```python
from build123d import *

# Parameters (mm, degrees)
F1_DEPTH = 203.2
F2_R     = 3.69316
F3_R     = 1.98374
F4_R     = 0.762
F5_R     = 1.35255
F6_DEPTH = 1.70942


with BuildPart() as f1:
    # F0 (on Top) → F1 (new body)
    with BuildSketch(Plane.XY):
        Polygon((0, -34.912743), (0, 0), (4.632677, 3.932751), (7.97125, 0), (9.274422, 1.106282), (4.829567, 6.342205), (-1.70942, 0.791159), (-1.70942, -36.622163), (155.970525, -36.622163), (155.970525, 0.791159), (149.431538, 6.342205), (144.986683, 1.106282), (146.289855, 0), (149.628427, 3.932751), (154.261105, 0), (154.261105, -34.912743), align=None)
    extrude(amount=F1_DEPTH)

    # F2
    f2_edges = [f1.edges().sort_by_distance(p)[0] for p in [
        (149.431538, 6.342205, 101.6),
        (155.970525, 0.791159, 101.6),
        (155.970525, -36.622163, 101.6),
        (-1.70942, -36.622163, 101.6),
        (-1.70942, 0.791159, 101.6),
        (4.829567, 6.342205, 101.6),
    ]]
    fillet(f2_edges, radius=F2_R)

    # F3
    f3_edges = [f1.edges().sort_by_distance(p)[0] for p in [
        (149.628427, 3.932751, 101.6),
        (154.261105, 0, 101.6),
        (154.261105, -34.912743, 101.6),
        (0, -34.912743, 101.6),
        (0, 0, 101.6),
        (4.632677, 3.932751, 101.6),
    ]]
    fillet(f3_edges, radius=F3_R)

    # F4
    f4_edges = [f1.edges().sort_by_distance(p)[0] for p in [
        (145.638269, 0.553141, 203.2),
        (145.638269, 0.553141, 0),
        (8.622836, 0.553141, 0),
        (8.622836, 0.553141, 203.2),
    ]]
    fillet(f4_edges, radius=F4_R)

    # F5 (on face) → F6 (cut, through all)
    with BuildSketch(Plane(origin=(0, -34.912743, 0), x_dir=(-1, 0, 0), z_dir=(0, 1, 0))):
        with Locations((-5.15874, 3.175)):
            Circle(F5_R)
        with Locations((-5.15874, 101.6)):
            Circle(F5_R)
        with Locations((-5.15874, 200.025)):
            Circle(F5_R)
        with Locations((-149.102365, 200.025)):
            Circle(F5_R)
        with Locations((-149.102365, 101.6)):
            Circle(F5_R)
        with Locations((-149.102365, 3.175)):
            Circle(F5_R)
    extrude(amount=-F6_DEPTH, mode=Mode.SUBTRACT)


solid = f1.part
```
Here's how the part is built. I have some questions about the finished solid (model axes, mm). A direction names the side the tool comes from. Coordinates: 2 decimals unless noted, no trailing zeros. Loops run counter-clockwise (first coordinate to the right, second up) from the corner with the lowest first, then second, coordinate; pieces in that order, holes last. Notation, with made-up numbers: (3.5, 67.5) -> (12.5, 67.5) arc R19 ccw to (12.5, 101.5) -> close; hole circle Ø9 at (15.5, 13). An arc over 180 degrees is marked (long way). Return JSON: item names as keys, results as strings.
1) Thinking about a two-plate mould opening in X: for faces 3 (the face through (155.971, -17, 100)), 4 (the face through (76, -36.622, 100)), 5 (the face through (154.261, -17, 100)), which applies, +X half, -X half, draft (parallel to the pull), parting line (faces both ways), or undercut?
Results below:
{"face 3": "+X half", "face 4": "draft", "face 5": "undercut"}
2) If we section it at A-A, the plane y = -20.5: Write out the boundary of the cut face in (x, z).
Results below:
{"outline": "(-1.71, 0) -> (0, 0) -> (0, 203.2) -> (-1.71, 203.2) -> close; (154.26, 0) -> (155.97, 0) -> (155.97, 203.2) -> (154.26, 203.2) -> close"}
3) If we section it at C-C, the plane x = 92: Write out the boundary of the cut face in (y, z).
Results below:
{"outline": "(-36.62, 0) -> (-34.91, 0) -> (-34.91, 203.2) -> (-36.62, 203.2) -> close"}
4) For faces 1 (the face through (0, -17, 100)), 2 (the face through (4.745, 4.814, 103.022)), which set-ups out of +Z, -Z, +X, -X, +Y, -Y let a thin tool reach every point of the face, with its end or its side?
Results below:
{"face 1": "+Z, -Z", "face 2": "+Z, -Z, +Y"}
5) I need wall thicknesses on line 1 (X direction, y = -7, z = 99); line 2 (X direction, y = 2, z = 70); line 3 (X direction, y = -35.7, z = 101.6). Which ranges of each line are inside material? Lowest first, please. Write a range as from..to.
Results below:
{"line 1": "-1.71..0, 154.26..155.97", "line 2": "-0.29..2.36, 6.27..8.52, 145.75..147.99, 151.91..154.55", "line 3": "-0.46..3.81, 6.51..147.75, 150.45..154.72"}
6) If we section it at B-B, the plane z = 134: Write out the boundary of the cut face in (x, y), then the cut area to 3 significant figures.
Results below:
{"outline": "(-1.71, -32.93) arc R3.69 ccw to (1.98, -36.62) -> (152.28, -36.62) arc R3.69 ccw to (155.97, -32.93) -> (155.97, -0.92) arc R3.69 ccw to (154.67, 1.9) -> (152.25, 3.95) arc R3.69 ccw to (147.04, 3.53) -> (144.99, 1.11) -> (146.29, 0) -> (148.34, 2.42) arc R1.98 cw to (151.14, 2.65) -> (153.56, 0.59) arc R1.98 cw to (154.26, -0.92) -> (154.26, -32.93) arc R1.98 cw to (152.28, -34.91) -> (1.98, -34.91) arc R1.98 cw to (0, -32.93) -> (0, -0.92) arc R1.98 cw to (0.7, 0.59) -> (3.12, 2.65) arc R1.98 cw to (5.92, 2.42) -> (7.97, 0) -> (9.27, 1.11) -> (7.22, 3.53) arc R3.69 ccw to (2.01, 3.95) -> (-0.41, 1.9) arc R3.69 ccw to (-1.71, -0.92) -> close", "area": "427 mm²"}
